from build123d import *

# Parameters (mm, degrees)
F3_DEPTH = 150
F5_W     = 287.4648571014
F5_H     = 39.5074803382
F6_DEPTH = 100


with BuildPart() as f3:
    # F2 (on offset) → F3 (new body)
    with BuildSketch(Plane.YZ.offset(150)):
        with BuildLine():
            Line((75, 30), (-75, 30))
            add(Edge.make_bspline(
                [(-75, 30), (-71.9329359938, 17.6180406035), (-65.4869883967, -11.7202689141), (-24.2230739874, -0.0289004303), (-0.310510428, 0)],
                knots=[0, 0, 0, 0, 0.2139055177, 0.4987670748, 0.4987670748, 0.4987670748, 0.4987670748], degree=3))
            Line((-0.310510428, 0), (0, 0))
            add(Edge.make_bspline(
                [(0, 0), (24.0188569043, -0.0291511428), (66.5209416521, -11.9529873249), (70.3629883157, 17.8901810125), (75, 30)],
                knots=[0.5, 0.5, 0.5, 0.5, 0.7860944823, 1, 1, 1, 1], degree=3))
        make_face()
    extrude(amount=-F3_DEPTH)

    # F4: sweep along a path in F0
    with BuildLine(Plane.XZ) as f4_path:
        ThreePointArc((-115, 30), (-58.5173093171, 11.1003142846), (0, 0))
    # F3_face (on face) → F4 (sweep)
    with BuildSketch(Plane(origin=(0, -0.2555367718, 14.7206073646), x_dir=(0, 1, 0), z_dir=(-1, 0, 0))):
        with BuildLine():
            add(Edge.make_bspline(
                [(0.2555367718, 14.7206073646), (24.274393676, 14.7497585074), (66.7764784238, 26.6735946895), (70.6185250874, -3.1695736479), (75.2555367718, -15.2793926354)],
                knots=[0.5, 0.5, 0.5, 0.5, 0.7860944823, 1, 1, 1, 1], degree=3))
            Line((0.2555367718, 14.7206073646), (-0.0549736563, 14.7206073646))
            add(Edge.make_bspline(
                [(-74.7444632282, -15.2793926354), (-71.677399222, -2.8974332389), (-65.231451625, 26.4408762787), (-23.9675372157, 14.7495077949), (-0.0549736563, 14.7206073646)],
                knots=[0, 0, 0, 0, 0.2139055177, 0.4987670748, 0.4987670748, 0.4987670748, 0.4987670748], degree=3))
            Line((-74.7444632282, -15.2793926354), (75.2555367718, -15.2793926354))
        make_face()
    sweep(path=f4_path.line)

    # F5 (on Front) → F6 (cut, symmetric)
    with BuildSketch(Plane.XZ):
        with Locations((11.0934823751, 48.3694141731)):
            Rectangle(F5_W, F5_H)
    extrude(amount=F6_DEPTH, both=True, mode=Mode.SUBTRACT)


solid = f3.part
Source: CAD feature listing. Evaluate the final solid. Frame: model axes, mm. A direction names the side the tool comes from. Round coordinates to 2 decimals unless told otherwise and drop trailing zeros. Use a Markdown table: item, result. Add a question column.
1. First-contact query: pin 1 (1.5 mm diameter, centred on x = 107.5, z = 20, fed in from -Y); pin 2 (5 mm diameter, centred on x = -78, z = 23.5, fed in from +Y); pin 3 (5 mm diameter, centred on x = -39.5, z = 12.5, fed in from -Y). Flat tips, straight axial feed; report the tip coordinate or a pass-through.
2. Line query: probe 1 along Y at (x, z) = (-7, 3); probe 2 along Z at (x, y) = (61, -53.5); probe 3 along Z at (x, y) = (64, 27). Output: solid intervals per line, ascending.
3. Set-up query: faces 1 (the flat face through (150, -1, 13)), 2 (the cylindrical face through (-57.52, -0.16, 10.84)). Return all of +Z, -Z, +X, -X, +Y, -Y with unobstructed straight access to the full face (end or side cutting, diameter ignored); none if empty.
Derived:
| question | item | result |
|---|---|---|
| 1 | pin 1 | y = -72.64 |
| 1 | pin 2 | y = 67.62 |
| 1 | pin 3 | y = -67.91 |
| 2 | probe 1 | -63 to 62.78 |
| 2 | probe 2 | -2.24 to 28.62 |
| 2 | probe 3 | -1.87 to 28.62 |
| 3 | face 1 | +Z, -Z, +X, +Y, -Y |
| 3 | face 2 | -Z, -X |
